Drawing for the job (mm, zero at the part's lowest x, y, z). Give positions to 0.01 mm unless a question says otherwise; leave off trailing zeros. Write each loop counter-clockwise with the first axis right and the second up, starting at its lowest first coordinate (ties: lowest second). Pieces come first, ordered by that corner, then holes. Notation, with made-up numbers: (-23.5, 37) - (33.5, 37) arc R18 ccw to (33.5, 66) - close; hole circle Ø2 at (17.25, 29.5). An arc over 180 degrees is marked (long way). Answer as a JSON object with one key per item and string values. Group by question number.
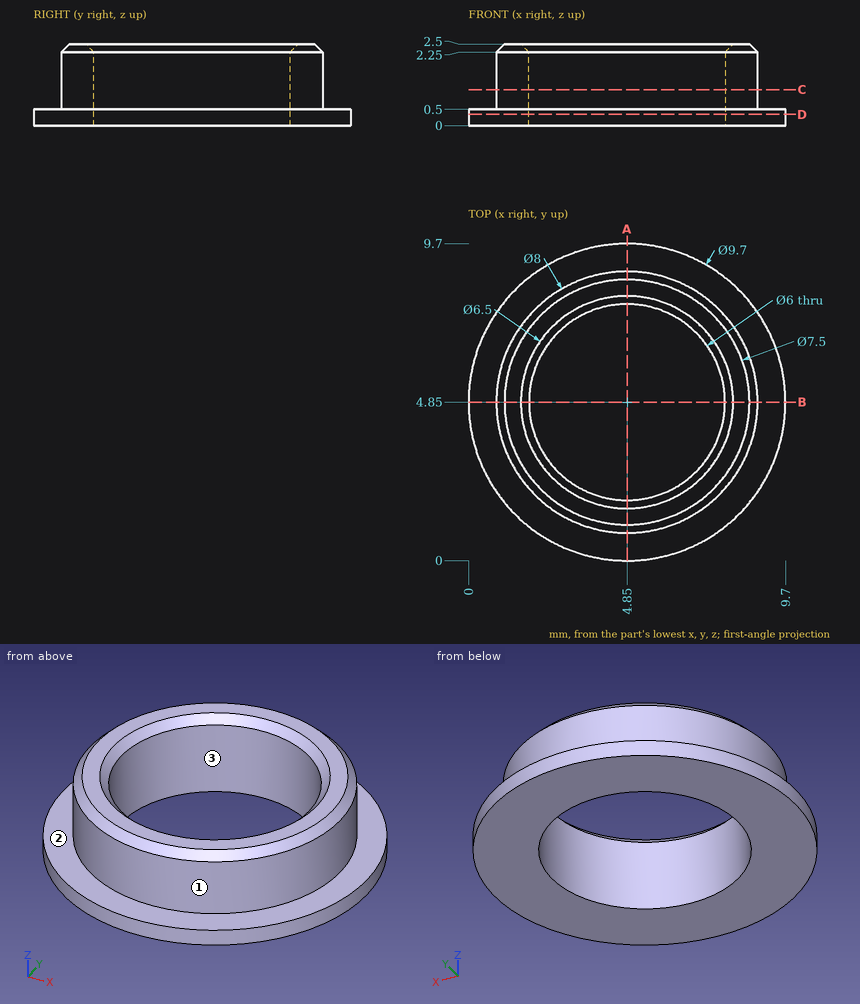
1) Band-saw the part on C-C (z = 1.1). List the corners of the cut face in (x, y), plus the area to 3 significant figures.
2) Probe line 1 (Y direction, x = 4.85, z = 1.5); line 2 (Y direction, x = 6, z = 1.45); line 3 (X direction, y = 7.25, z = 0.55). List the from-to ranges inside material, lowest first.
3) Band-saw the part on A-A (x = 4.85). List the corners of the cut face in (y, z).
4) Band-saw the part on D-D (z = 0.35). List the corners of the cut face in (x, y), plus the area to 3 significant figures.
5) Mould opens along Y. For the marked faces 1, 2 and 3 say: pulls with the +Y half, pulls with the -Y half, needs draft (parallel to the pull), parting line crosses it, or undercut.
6) Drop flat-ended pins along their axis: P1, Ø1, axis at x = 3.5, z = 1.5, coming from the +Y side; P2, Ø3, axis at x = 3.5, y = 4.5, coming from the +Z side; P3, Ø1.5, axis at x = 8.5, y = 1.5, coming from the +Z side. Give the stop position or say it passes through.
Verdict:
{
 "1": {"outline": "circle Ø8 at (4.85, 4.85); hole circle Ø6 at (4.85, 4.85)", "area": "22.0 mm2"},
 "2": {"line 1": "0.85 to 1.85, 7.85 to 8.85", "line 2": "1.02 to 2.08, 7.62 to 8.68", "line 3": "1.65 to 3.05, 6.65 to 8.05"},
 "3": {"outline": "(0, 0) - (1.85, 0) - (1.85, 2.25) - (1.6, 2.5) - (1.1, 2.5) - (0.85, 2.25) - (0.85, 0.5) - (0, 0.5) - close; (7.85, 0) - (9.7, 0) - (9.7, 0.5) - (8.85, 0.5) - (8.85, 2.25) - (8.6, 2.5) - (8.1, 2.5) - (7.85, 2.25) - close"},
 "4": {"outline": "circle Ø9.7 at (4.85, 4.85); hole circle Ø6 at (4.85, 4.85)", "area": "45.6 mm2"},
 "5": {"face 1": "parting line crosses it", "face 2": "needs draft", "face 3": "undercut"},
 "6": {"P1": "y = 8.76", "P2": "through", "P3": "z = 0.5"}
}
